Verification items for this drawing (mm, ordinates from the low corner). A direction names the side the tool comes from. Round coordinates to 2 decimals unless told otherwise and drop trailing zeros. Loops run counter-clockwise (first coordinate to the right, second up) from the corner with the lowest first, then second, coordinate; pieces in that order, holes last. Notation, with made-up numbers: (-35, 0.25) - (-21, 0.25) arc R31 ccw to (-21, 32.25) - close; hole circle Ø3 at (-31.75, 71). An arc over 180 degrees is marked (long way). Answer in a Markdown table with one row per item. Add a question column.
(1) Cross-section at A-A on z = 2.5. Enter the section's corners in (x, y), then the cut area to 3 significant figures.
(2) Gauge pin test, flat ends, axial feed: pin 1 (1.8 mm diameter, centred on y = 15, z = 3.5, fed in from +X); pin 2 (3 mm diameter, centred on x = 26.5, z = 3.5, fed in from +Y); pin 3 (1.1 mm diameter, centred on y = 25, z = 4, fed in from -X). Record the tip position at first contact, or that the pin passes through.
(3) Cross-section at B-B on x = 27.07. Enter the section's corners in (y, z).
(4) Thickness scan on line 1 along Y through (x, z) = (16.31, 0.4); line 2 along X through (y, z) = (14, 1.3); line 3 along X through (y, z) = (13, 3). Record the ranges inside material, lowest first.
(5) Cross-section at D-D on x = 16.31. Enter the section's corners in (y, z), then the cut area to 3 significant figures.
(6) Access from +Z, -Z, +X, -X, +Y, -Y to the whole of each face (thin tool, end or side, straight path). Record for the marked faces 1, 2, 3, 4 and 5.
(7) Cross-section at C-C on y = 14. Enter the section's corners in (x, z).
(8) Mould release check, pull along Y, two halves, no side actions. Record for the marked faces 6, 7 and 8: +Y half, -Y half, draft (parallel to the pull), parting line (faces both ways), or undercut.
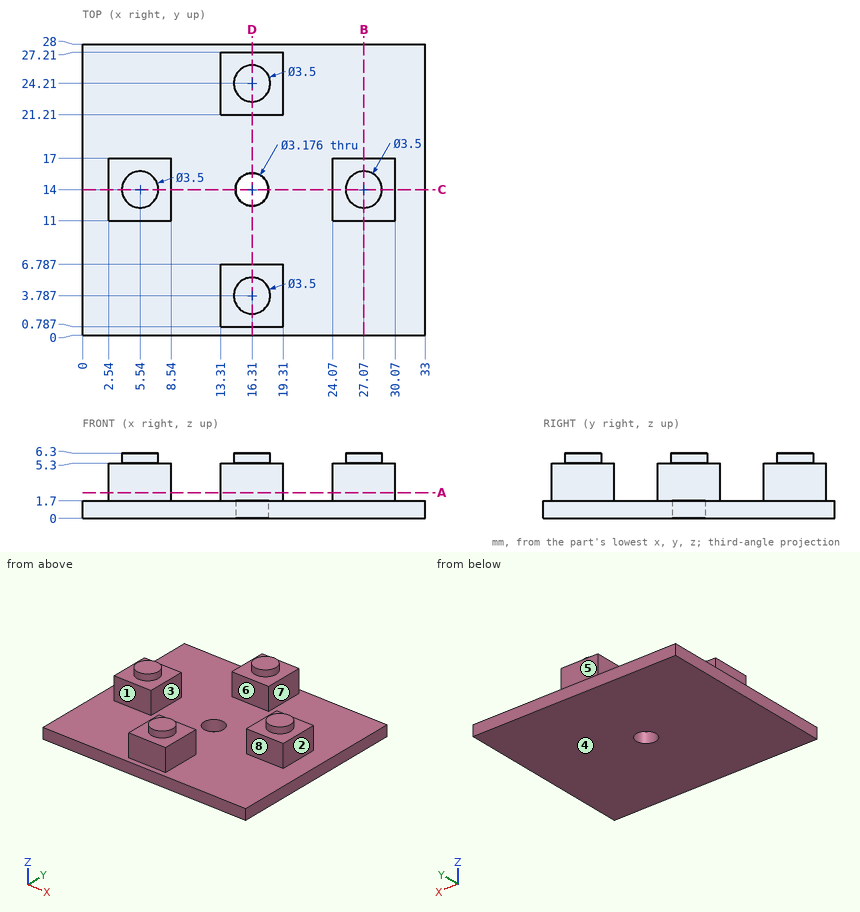
Answers:
| question | item | result |
|---|---|---|
| 1 | outline | (2.54, 11) - (8.54, 11) - (8.54, 17) - (2.54, 17) - close; (13.31, 0.79) - (19.31, 0.79) - (19.31, 6.79) - (13.31, 6.79) - close; (13.31, 21.21) - (19.31, 21.21) - (19.31, 27.21) - (13.31, 27.21) - close; (24.07, 11) - (30.07, 11) - (30.07, 17) - (24.07, 17) - close |
| 1 | area | 144 mm^2 |
| 2 | pin 1 | stops at x = 30.07 |
| 2 | pin 2 | stops at y = 17 |
| 2 | pin 3 | stops at x = 13.31 |
| 3 | outline | (0, 0) - (28, 0) - (28, 1.7) - (17, 1.7) - (17, 5.3) - (15.75, 5.3) - (15.75, 6.3) - (12.25, 6.3) - (12.25, 5.3) - (11, 5.3) - (11, 1.7) - (0, 1.7) - close |
| 4 | line 1 | y = 0 to 12.41, 15.59 to 28 |
| 4 | line 2 | x = 0 to 14.72, 17.9 to 33 |
| 4 | line 3 | x = 2.54 to 8.54, 24.07 to 30.07 |
| 5 | outline | (0, 0) - (12.41, 0) - (12.41, 1.7) - (6.79, 1.7) - (6.79, 5.3) - (5.54, 5.3) - (5.54, 6.3) - (2.04, 6.3) - (2.04, 5.3) - (0.79, 5.3) - (0.79, 1.7) - (0, 1.7) - close; (15.59, 0) - (28, 0) - (28, 1.7) - (27.21, 1.7) - (27.21, 5.3) - (25.96, 5.3) - (25.96, 6.3) - (22.46, 6.3) - (22.46, 5.3) - (21.21, 5.3) - (21.21, 1.7) - (15.59, 1.7) - close |
| 5 | area | 92.4 mm^2 |
| 6 | face 1 | +Z, +X, -X, -Y |
| 6 | face 2 | +Z, +X, +Y, -Y |
| 6 | face 3 | +Z, +Y, -Y |
| 6 | face 4 | -Z, +X, -X, +Y, -Y |
| 6 | face 5 | +Z, +X, -X, +Y |
| 7 | outline | (0, 0) - (14.72, 0) - (14.72, 1.7) - (8.54, 1.7) - (8.54, 5.3) - (7.29, 5.3) - (7.29, 6.3) - (3.79, 6.3) - (3.79, 5.3) - (2.54, 5.3) - (2.54, 1.7) - (0, 1.7) - close; (17.9, 0) - (33, 0) - (33, 1.7) - (30.07, 1.7) - (30.07, 5.3) - (28.82, 5.3) - (28.82, 6.3) - (25.32, 6.3) - (25.32, 5.3) - (24.07, 5.3) - (24.07, 1.7) - (17.9, 1.7) - close |
| 8 | face 6 | undercut |
| 8 | face 7 | draft |
| 8 | face 8 | -Y half |
